Autodesk Inventor part; units mm, degrees
ref_plane "Work Plane3" through (-3.175, -2.433, 10) normal (-1, 0, 0) x (0, 0, 1)
ref_plane "YZ Plane" through (0, 0, 0) normal (1, 0, 0) x (0, 1, 0)
ref_plane "XZ Plane" through (0, 0, 0) normal (0, 1, 0) x (-1, 0, 0)
sketch "Sketch1" plane through (0, 0, 0) normal (0, 0, 1) x (1, 0, 0)
  circle A0 centre (0, 0) radius 6
  line L0 (-7.6, 2) -> (-5.6569, 2)
  line L1 (-7.6, 2) -> (-7.6, -2)
  line L2 (-5.6569, -2) -> (-7.6, -2)
  circle A1 centre (0, 0) radius 12.5
  point P0 (0, 0)
  dimension "d0" = 25
extrude "Extrusion1" add sketch "Sketch1" against normal blind 14
sketch "Sketch2" plane through (0, 0, 0) normal (0, 0, 1) x (1, 0, 0)
  arc A0 (19.4059, 4.8385) -> (16.8372, 10.794) centre (0, 0) ccw
  circle A1 centre (0, 0) radius 12.5
  point P0 (0, 0)
extrude "Extrusion2" add sketch "Sketch2" along normal blind 8
sketch "Sketch3" plane through (0, 0, 8) normal (0, 0, 1) x (1, 0, 0)
  circle A0 centre (0, 0) radius 12.5
  line L0 (-3.175, -2.433) -> (-3.175, 2.433)
  arc A1 (-3.175, -2.433) -> (-3.175, 2.433) centre (0, 0) ccw
  point P0 (0, 0)
extrude "Extrusion3" add sketch "Sketch3" along normal blind 12
ref_plane "Work Plane2" through (-12.5, 0, 0) normal (-1, 0, 0) x (0, -1, 0)
ref_plane "Work Plane1" through (-3.175, -2.433, 10) normal (-1, 0, 0) x (0, 1, 0)
sketch "Sketch4" plane through (-12.5, 0, 0) normal (-1, 0, 0) x (0, -1, 0)
  circle A0 centre (0, 12) radius 3
  line L0 (12.5, 20) -> (-12.5, 20)
  point P0 (0, 0)
  dimension "d7" = 8
  dimension "d8" = 6
ref_plane "Work Plane3" through (-3.175, -2.433, 10) normal (-1, 0, 0) x (0, 0, 1)
extrude "Extrusion4" cut sketch "Sketch4" against normal up to surface (9.325 mm away)
thread "Thread1"
properties part number "nmrv-50 to megatroque motor coupler"
Input: part model. Units: mm. Frame: model coordinates. A direction names the side the tool comes from. Coordinates: 2 decimals unless noted, no trailing zeros. Loops run counter-clockwise (first coordinate to the right, second up) from the corner with the lowest first, then second, coordinate; pieces in that order, holes last. Notation, with made-up numbers: M 37,37 L 58,37 A28 cw 58,68 Z; hole C 1,72.25 d6. An arc over 180 degrees is marked long. One line per item, written item: value.
(1) Section B-B (x = 0). Output: boundary loops of the cut face in (y, z).
Filled in:
outline: M -12.5,-14 L -6,-14 L -6,0 L 6,0 L 6,-14 L 12.5,-14 L 12.5,20 L 4,20 L 4,8 L -4,8 L -4,20 L -12.5,20 Z
(2) Section C-C (z = -3). Output: boundary loops of the cut face in (x, y).
Filled in:
outline: C 0,0 d25; hole M -7.6,-2 L -5.66,-2 A6 ccw long -5.66,2 L -7.6,2 Z
(3) Pull-direction query (X, two-part tool) for faces 4 (the cylindrical face through (11.923, -3.755, 2.762)), 5 (the cylindrical face through (-7.9, 0.65, 9.07)), 6 (the cylindrical face through (4, 0, 14)); classes: +X half, -X half, draft (parallel to the pull), parting line (faces both ways), or undercut.
Filled in:
face 4: parting line
face 5: draft
face 6: undercut
(4) Pin query (flat end, axial travel): pin 1 (1.5 mm diameter, centred on y = 3.5, z = 15.5, fed in from -X); pin 2 (5 mm diameter, centred on x = 0, y = 0, fed in from +Z); pin 3 (1.6 mm diameter, centred on x = -7, z = -4, fed in from -Y). Return the tip coordinate at first contact, or that it passes through.
Filled in:
pin 1: x = -12.19
pin 2: z = 8
pin 3: y = -10.85
(5) Reachability of faces 1 (the flat face through (-3, -5.4, -14)), 2 (the flat face through (-7, 2, -7)), 3 (the flat face through (-3.175, 0, 18)) from +Z, -Z, +X, -X, +Y, -Y: full face, straight path, thin tool, end or side. Return the list, or none.
Filled in:
face 1: -Z, +X, -X, +Y, -Y
face 2: -Z
face 3: +Z
(6) Section D-D (x = -4.25). Output: boundary loops of the cut face in (y, z), and give its area (4 significant figures).
Filled in:
outline: M -11.76,-14 L -4.24,-14 L -4.24,0 L 4.24,0 L 4.24,-14 L 11.76,-14 L 11.76,20 L -11.76,20 Z; hole C 0,12 d6
area: 652.5 mm^2
(7) Line query: line 1 along Z through (x, y) = (-6.25, 0); line 2 along Y through (x, z) = (0, -9); line 3 along Y through (x, z) = (0, 16). Output: solid intervals per line, ascending. Write a range as from..to.
Filled in:
line 1: 0..9, 15..20
line 2: -12.5..-6, 6..12.5
line 3: -12.5..-4, 4..12.5
(8) Section A-A (y = 0). Output: boundary loops of the cut face in (x, z) (3 decimals).
Filled in:
outline: M -12.5,-14 L -7.6,-14 L -7.6,0 L 6,0 L 6,-14 L 12.5,-14 L 12.5,20 L 4,20 L 4,8 L -3.175,8 L -3.175,9 L -12.5,9 Z; M -12.5,15 L -3.175,15 L -3.175,20 L -12.5,20 Z
